Design review of the part built by this model. Coordinates are the model's own, in mm. Give positions to 0.01 mm unless a question says otherwise; leave off trailing zeros. Loops run counter-clockwise (first coordinate to the right, second up) from the corner with the lowest first, then second, coordinate; pieces in that order, holes last. Notation, with made-up numbers: (-12, 40) - (-8, 40) arc R26 ccw to (-8, 69) - close; hole circle Ø8 at (57, -30). An arc over 180 degrees is marked (long way). One line per item, written item: value. Start each with the question number.
Autodesk Inventor part; units mm, degrees
ref_plane "YZ Plane" through (0, 0, 0) normal (1, 0, 0) x (0, 1, 0)
ref_plane "XZ Plane" through (0, 0, 0) normal (0, 1, 0) x (-1, 0, 0)
ref_plane "XY Plane" through (0, 0, 0) normal (0, 0, 1) x (1, 0, 0)
sketch "Sketch1" plane through (0, 0, 0) normal (0, 0, 1) x (1, 0, 0)
  line L0 (0, 3.75) -> (2, 3.75)
  line L1 (2, 3.75) -> (2, -4)
  line L2 (2, -4) -> (0, -4)
  line L3 (0, -4) -> (0, 3.75) construction
  line L4 (0, -4) -> (-5, -4)
  line L5 (-5, -4) -> (-5, -1)
  line L6 (-5, -1) -> (0, -1)
  line L7 (0, 3.75) -> (-1, 3.75)
  line L8 (-1, 3.75) -> (-1, 0.75)
  line L9 (-1, 0.75) -> (0, 0.75)
  line L10 (0, 0.75) -> (0, 3.75) construction
  line L11 (0, 0.75) -> (0, -1)
  point P0 (0, 0)
  point P1 (0, -0.125)
  point P2 (1, 3.75)
  dimension "d0" = 4
  dimension "d1" = 2
  dimension "d5" = 5
  dimension "d6" = 1.75
  dimension "d7" = 3
  dimension "d11" = 3
  dimension "d12" = 3
extrude "Extrusion1" add sketch "Sketch1" along normal blind 245.505
sketch "Sketch2" plane through (-1, 3.75, 245.505) normal (0, 1, 0) x (1, 0, 0)
  line L0 (3, 245.505) -> (3, 0) construction
  line L1 (3, 122.7525) -> (1, 122.7525) construction
  line L2 (1, 245.505) -> (1, 0) construction
  line L3 (3, 127.3525) -> (1, 127.3525)
  line L4 (1, 127.3525) -> (1, 118.1525) construction
  line L5 (1, 118.1525) -> (3, 118.1525) construction
  line L6 (3, 118.1525) -> (3, 127.3525)
  line L7 (3, 122.7525) -> (1, 122.7525) construction
  line L8 (3, 118.1525) -> (1, 118.1525)
  line L9 (1, 127.3525) -> (0, 127.3525)
  line L10 (0, 245.505) -> (0, 0)
  line L11 (0, 127.3525) -> (0, 118.1525)
  line L12 (0, 118.1525) -> (1, 118.1525)
  point P0 (0, 118.1525)
  dimension "d13" = 9.2
extrude "Extrusion2" cut sketch "Sketch2" against normal up to surface (3 mm away)
sketch "Sketch3" plane through (-1, 0.75, 0) normal (-1, 0, 0) x (0, 0, 1)
  line L0 (118.1525, 0) -> (118.1525, 3)
  line L1 (0, 3) -> (118.1525, 3)
  line L2 (0, 3) -> (0, 0)
  line L3 (0, 0) -> (118.1525, 0)
  line L4 (127.3525, 3) -> (127.3525, 0)
  line L5 (127.3525, 0) -> (245.505, 0)
  line L6 (245.505, 3) -> (245.505, 0)
  line L7 (127.3525, 3) -> (245.505, 3)
  point P0 (0, -0.75)
extrude "Extrusion3" cut sketch "Sketch3" against normal blind 0.9
chamfer "Chamfer1" distance 2.5 angle 45 1 edges at (-5, -4, 122.7525)
sketch "Sketch4" plane through (-0.1, 0.75, 0) normal (-1, 0, 0) x (0, 0, 1)
  line L0 (0, 3) -> (118.1525, 3)
  line L1 (0, 3) -> (2.45, 3)
  line L2 (2.45, 3) -> (2.45, 0.55)
  line L3 (2.45, 0.55) -> (0, 0.55)
  line L4 (0, 0.55) -> (0, 3)
  line L5 (127.3525, 3) -> (245.505, 3)
  line L6 (245.505, 3) -> (243.055, 3)
  line L7 (243.055, 3) -> (243.055, 0.55)
  line L8 (243.055, 0.55) -> (245.505, 0.55)
  line L9 (245.505, 0.55) -> (245.505, 3)
  line L10 (0, 3) -> (2.45, 3)
  line L11 (2.45, 3) -> (2.45, 0.55)
  line L12 (245.505, 3) -> (243.055, 3)
  line L13 (243.055, 3) -> (243.055, 0.55)
  point P0 (0, -0.75)
  dimension "d21" = 2.45
  dimension "d22" = 2.45
  dimension "d23" = 2.45
  dimension "d24" = 2.45
extrude "Extrusion4" add sketch "Sketch4" along normal blind 2.95
sketch "Sketch5" plane through (-0.1, 0.75, 0) normal (-1, 0, 0) x (0, 0, 1)
  line L0 (114.505, 2.85) -> (114.505, 0.85) construction
  line L1 (131, 0.85) -> (131, 2.85) construction
  line L2 (131, 2.85) -> (131, 3) construction
  line L3 (127.3525, 3) -> (243.055, 3) construction
  line L4 (114.505, 2.85) -> (114.505, 3) construction
  line L5 (114.505, 3) -> (117.005, 3)
  line L6 (117.005, 3) -> (117.005, 1.05)
  line L7 (117.005, 1.05) -> (114.505, 1.05)
  line L8 (114.505, 1.05) -> (114.505, 3)
  line L9 (131, 3) -> (128.5, 3)
  line L10 (128.5, 3) -> (128.5, 1.05)
  line L11 (128.5, 1.05) -> (131, 1.05)
  line L12 (131, 1.05) -> (131, 3)
  line L13 (2.45, 3) -> (118.1525, 3)
  point P0 (0, -0.75)
  dimension "d27" = 2.5
  dimension "d28" = 2.5
  dimension "d29" = 1.95
extrude "Extrusion5" add sketch "Sketch5" along normal blind 2.95
sketch "Sketch6" plane through (-0.1, 0.75, 0) normal (-1, 0, 0) x (0, 0, 1)
  line L0 (172.5025, 2.85) -> (172.5025, 0.85) construction
  line L1 (177.6025, 0.85) -> (177.6025, 2.85) construction
  line L2 (177.6025, 2.85) -> (177.6025, 3) construction
  line L3 (131, 3) -> (243.055, 3) construction
  line L4 (172.5025, 2.85) -> (172.5025, 3) construction
  line L5 (172.7025, 3) -> (177.4025, 3)
  line L6 (177.4025, 3) -> (177.4025, 1.05)
  line L7 (177.4025, 1.05) -> (172.7025, 1.05)
  line L8 (172.7025, 1.05) -> (172.7025, 3)
  point P0 (0, -0.75)
  dimension "d32" = 0.2
  dimension "d33" = 0.2
  dimension "d34" = 1.95
extrude "Extrusion6" add sketch "Sketch6" along normal blind 2.95
properties part number "Top Case Rail" material "PET Plastic"
(1) To check wall thickness, follow L1, parallel to Z at x = 1, y = 2.5 (1 decimal); L2, parallel to Z at x = -3, y = 1.5 (3 decimals); L3, parallel to X at y = 2.5, z = 22.5. State the ranges of each line that lie inside material, in increasing order. Write a range as from..to.
(2) Take a section at A-A on x = -1.25. State how many separate pieces and enclosed holes the cut face has, and give its area (3 significant figures).
(3) Take a section at B-B on z = 151.5. State the section outline as (x, y) points, and give its area (3 significant figures).
(4) For pin 1 Ø0.6 at (x, z) = (1.5, 122) entering from +Y; pin 2 Ø1.6 at (y, z) = (2.5, 129.5) entering from -X; pin 3 Ø4 at (x, z) = (-2.5, 81.5) entering from +Y, all flat-tipped, find the tip position at first contact; note any pin that passes through.
Here are the results:
1. L1: 0..118.2, 127.4..245.5
1. L2: 0..2.45, 243.055..245.505
1. L3: -0.1..2
2. separate pieces: 6
2. enclosed holes: 0
2. area: 767 mm²
3. outline: (-5, -1.5) - (-2.5, -4) - (2, -4) - (2, 3.75) - (-0.1, 3.75) - (-0.1, 0.75) - (0, 0.75) - (0, -1) - (-5, -1) - close
3. area: 27.7 mm²
4. pin 1: y = 0.75
4. pin 2: x = -3.05
4. pin 3: y = -1
